Source: CAD feature listing. Evaluate the final solid. Frame: model axes, mm. A direction names the side the tool comes from. Coordinates: 2 decimals unless noted, no trailing zeros. Order: outer loops, then holes, each group sorted by start corner. A loop starts at its lowest first (then second) coordinate and runs counter-clockwise, first axis right, second up.
```python
from build123d import *

# Parameters (mm, degrees)
SKETCH1_R           = 2.5
SKETCH1_R_2         = 1.5
BOSS_EXTRUDE1_DEPTH = 4


with BuildPart() as part:
    # Sketch1 → Boss-Extrude1 (new body)
    with BuildSketch(Plane.XY):
        with BuildLine():
            Line((9.021718503, 2), (41.978281497, 2))
            ThreePointArc((41.978281497, 2), (44.822515117, 1.112217786), (46.656724728, -1.235865953))
            Line((46.656724728, -1.235865953), (46.789401092, -1.587720642))
            ThreePointArc((46.789401092, -1.587720642), (52.790694487, -4.128366899), (55.036357188, 1.989427216))
            Line((55.036357188, 1.989427216), (47.115238631, 18.060617738))
            ThreePointArc((47.115238631, 18.060617738), (43.216566444, 20.280145198), (39.708839684, 17.483397096))
            ThreePointArc((39.708839684, 17.483397096), (35.851166353, 12.07387553), (29.538291134, 10.002119376))
            Line((29.538291134, 10.002119376), (9.504810122, 10.002119376))
            ThreePointArc((9.504810122, 10.002119376), (4.286155076, 11.471841566), (0.601494655, 15.448991475))
            Line((0.601494655, 15.448991475), (-9.880645528, 35.94606576))
            ThreePointArc((-9.880645528, 35.94606576), (-10.802085001, 38.853975504), (-11.524402661, 41.817629833))
            ThreePointArc((-11.524402661, 41.817629833), (-13.960734342, 45.822125323), (-18.377595021, 47.391532194))
            Line((-18.377595021, 47.391532194), (-28.76016905, 47.391532194))
            ThreePointArc((-28.76016905, 47.391532194), (-30.76016905, 45.391532194), (-28.76016905, 43.391532194))
            Line((-28.76016905, 43.391532194), (-20.743770069, 43.391532194))
            ThreePointArc((-20.743770069, 43.391532194), (-17.93067591, 42.525114327), (-16.092507767, 40.226132695))
            ThreePointArc((-16.092507767, 40.226132695), (-15.696247775, 38.141532194), (-16.092507767, 36.056931692))
            ThreePointArc((-16.092507767, 36.056931692), (-17.93067591, 33.75795006), (-20.743770069, 32.891532194))
            Line((-20.743770069, 32.891532194), (-23.62255188, 32.891532194))
            Line((-23.62255188, 32.891532194), (-28.76016905, 32.891532194))
            ThreePointArc((-28.76016905, 32.891532194), (-30.76016905, 30.891532194), (-28.76016905, 28.891532194))
            Line((-28.76016905, 28.891532194), (-23.62255188, 28.891532194))
            ThreePointArc((-23.62255188, 28.891532194), (-18.403896833, 27.421810003), (-14.719236412, 23.444660095))
            Line((-14.719236412, 23.444660095), (-4.823396458, 4.094053908))
            ThreePointArc((-4.823396458, 4.094053908), (-4.495519345, 3.207734666), (-4.38472424, 2.269230727))
            Line((-4.38472424, 2.269230727), (-4.385851303, 1.007128763))
            ThreePointArc((-4.385851303, 1.007128763), (-1.300380409, -4.308017037), (4.210598908, -1.587720642))
            Line((4.210598908, -1.587720642), (4.343275272, -1.235865953))
            ThreePointArc((4.343275272, -1.235865953), (6.177484883, 1.112217786), (9.021718503, 2))
        make_face()
        Circle(SKETCH1_R, mode=Mode.SUBTRACT)
        with Locations((51, 0)):
            Circle(SKETCH1_R, mode=Mode.SUBTRACT)
        with Locations((43.150236609, 12)):
            Circle(SKETCH1_R_2, mode=Mode.SUBTRACT)
        with Locations((43.150236609, 16)):
            Circle(SKETCH1_R_2, mode=Mode.SUBTRACT)
    extrude(amount=BOSS_EXTRUDE1_DEPTH)


solid = part.part
```
1. Access query for faces 4 (the face through (20, 10.002, 2)), 5 (the face through (-26, 28.892, 2)), 6 (the face through (53.31, -0.96, 1.97)), 7 (the face through (-25, 43.392, 2)). Directions: +Z, -Z, +X, -X, +Y, -Y. A direction counts if a zero-diameter tool reaches every point of the face in a straight line with its end or side. Return the directions, or none.
Findings:
face 4: +Z, -Z, +Y
face 5: +Z, -Z, -X, -Y
face 6: +Z, -Z
face 7: +Z, -Z, -X
2. Section query C-C on y = 12. Return loops of the section in (x, z), plus the area to 3 significant figures.
Findings:
outline: (-8.87, 0) - (3.51, 0) - (3.51, 4) - (-8.87, 4) - close; (35.75, 0) - (41.65, 0) - (41.65, 4) - (35.75, 4) - close; (44.65, 0) - (50.1, 0) - (50.1, 4) - (44.65, 4) - close
area: 94.9 mm2
3. Section query B-B on y = 0. Return loops of the section in (x, z), plus the area to 3 significant figures.
Findings:
outline: (-4.5, 0) - (-2.5, 0) - (-2.5, 4) - (-4.5, 4) - close; (2.5, 0) - (5.02, 0) - (5.02, 4) - (2.5, 4) - close; (45.98, 0) - (48.5, 0) - (48.5, 4) - (45.98, 4) - close; (53.5, 0) - (55.5, 0) - (55.5, 4) - (53.5, 4) - close
area: 36.2 mm2
4. Section query D-D on x = 51. Return loops of the section in (y, z), plus the area to 3 significant figures.
Findings:
outline: (-4.5, 0) - (-2.5, 0) - (-2.5, 4) - (-4.5, 4) - close; (2.5, 0) - (10.18, 0) - (10.18, 4) - (2.5, 4) - close
area: 38.7 mm2
5. Section query A-A on z = 3.15. Count the separate pieces of the cut face and the enclosed holes in it, plus the area to 3 significant figures.
Findings:
separate pieces: 1
enclosed holes: 4
area: 1,080 mm2
6. Pin query (flat end, axial travel): P1, Ø4, axis at x = 43.15, y = 12, coming from the -Z side; P2, Ø2, axis at y = 1.5, z = 2.5, coming from the -X side; P3, Ø1, axis at x = -21, z = 3, coming from the -Y side; P4, Ø2, axis at x = -27, z = 2.5, coming from the -Y side. Return the tip coordinate at first contact, or that it passes through.
Findings:
P1: stops at z = 0
P2: stops at x = -4.47
P3: stops at y = 28.39
P4: stops at y = 28.89
7. Ray query, line 1 (Y direction, x = -23, z = 1.4); line 2 (Y direction, x = 20.5, z = 0.3); line 3 (Y direction, x = -17, z = 1.65). Return the intervals inside material, ascending.
Findings:
line 1: y = 28.87 to 32.89, 43.39 to 47.39
line 2: y = 2 to 10
line 3: y = 26.38 to 34.58, 41.71 to 47.25
8. Draft query along Y for faces 1 (the face through (-30.76, 45.44, 1.97)), 2 (the face through (35.93, 12.13, 1.97)), 3 (the face through (6, 8, 0)). Return one class per face: released by +Y, released by -Y, zero draft, split by the parting line, or undercut.
Findings:
face 1: undercut
face 2: released by +Y
face 3: zero draft
